Design review of the part built by this model. Coordinates are the model's own, in mm. Give positions to 0.01 mm unless a question says otherwise; leave off trailing zeros. Write each loop counter-clockwise with the first axis right and the second up, starting at its lowest first coordinate (ties: lowest second). Pieces come first, ordered by that corner, then holes. Notation, with made-up numbers: M 4.5,85 L 29.5,85 A13 cw 29.5,107 Z; hole C 60.25,54 d11. An arc over 180 degrees is marked long. Answer in a Markdown table with one row per item.
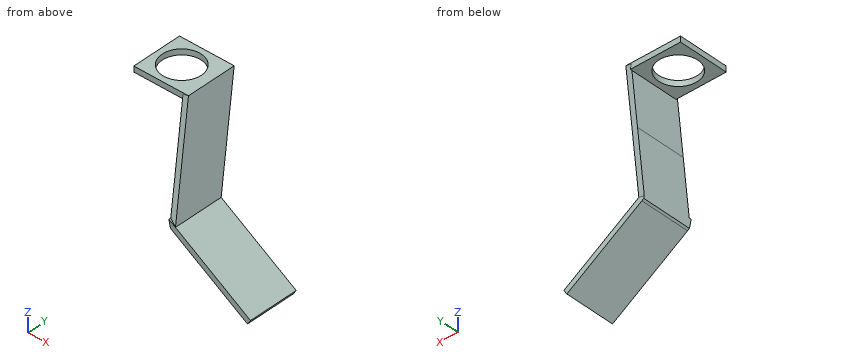
Autodesk Inventor part; units mm, degrees
ref_plane "YZ Plane" through (0, 0, 0) normal (1, 0, 0) x (0, 1, 0)
ref_plane "XZ Plane" through (0, 0, 0) normal (0, 1, 0) x (-1, 0, 0)
ref_plane "XY Plane" through (0, 0, 0) normal (0, 0, 1) x (1, 0, 0)
sketch "Sketch1" plane through (0, 0, 0) normal (0, 1, 0) x (-1, 0, 0)
  line L0 (43.0137, 64.3915) -> (32.1817, 14.8739)
  line L1 (-10.5502, -12.5966) -> (-8.8333, -15.2673)
  line L2 (-8.8333, -15.2673) -> (35.0028, 12.913)
  line L3 (35.0028, 12.913) -> (46.1153, 63.713)
  line L4 (46.1153, 63.713) -> (43.0137, 64.3915)
  line L5 (-10.5502, -12.5966) -> (-10.5502, 12.913)
  line L6 (-10.5502, -12.5966) -> (32.1817, 14.8739)
  line L7 (46.1153, 63.713) -> (74.6903, 63.713)
  line L8 (74.6903, 63.713) -> (74.6903, 66.888)
  line L9 (74.6903, 66.888) -> (43.5598, 66.888)
  line L10 (43.0137, 64.3915) -> (43.5598, 66.888)
  point P0 (0, 0)
  dimension "d0" = 3.175
  dimension "d1" = 3.175
  dimension "d3" = 50.8
  dimension "d4" = 57.265
  dimension "d5" = 50.8
  dimension "d6" = 11.1125
  dimension "d7" = 28.575
  dimension "d8" = 3.175
extrude "Extrusion1" add sketch "Sketch1" along normal blind 28.575
sketch "Sketch2" plane through (-74.6903, 0, 66.888) normal (0, 0, 1) x (1, 0, 0)
  line L0 (28.575, 0) -> (0, 0)
  line L1 (0, 0) -> (0, 28.575)
  line L2 (28.575, 28.575) -> (0, 28.575)
  line L3 (28.575, 0) -> (28.575, 28.575)
  line L4 (28.575, 28.575) -> (0, 28.575)
  line L5 (0, 0) -> (0, 28.575)
  circle A0 centre (14.2875, 14.2875) radius 11.1125
  point P0 (74.6903, 0)
  point P1 (14.2875, 28.575)
  point P2 (0, 14.2875)
  dimension "d11" = 22.225
extrude "Extrusion2" cut sketch "Sketch2" against normal blind 28.575 contours A0
sketch "Sketch3" plane through (10.5502, 0, -12.5966) normal (0.5408, 0, 0.8412) x (0.8412, 0, -0.5408)
  line L0 (-50.8, 0) -> (-50.8, 28.575)
  line L1 (-50.8, 7.9375) -> (0, 7.9375)
  line L2 (0, 7.9375) -> (0, -20.6375)
  line L3 (0, -20.6375) -> (-50.8, -20.6375)
  line L4 (-50.8, -20.6375) -> (-50.8, 7.9375)
  line L5 (-50.8, 28.575) -> (0, 28.575)
  point P0 (-15.6863, 0)
  dimension "d14" = 50.8
  dimension "d15" = 28.575
  dimension "d16" = 20.6375
sketch "Sketch4" plane through (-32.1817, 0, 14.8739) normal (0.9769, 0, 0.2137) x (0.2137, 0, -0.9769)
  line L0 (-53.2441, 0) -> (-53.2441, 28.575)
  line L1 (-53.2441, 28.575) -> (0, 7.9375)
  line L2 (0, 0) -> (0, 28.575)
  line L3 (0, 7.9375) -> (0, -20.6375)
  line L4 (0, -20.6375) -> (-53.2441, 0)
  line L5 (-53.2441, 28.575) -> (-53.2441, 0)
  point P0 (21.4074, 0)
  dimension "d17" = 20.6375
  dimension "d18" = 28.575
sketch "Sketch5" plane through (-32.1817, 0, 14.8739) normal (0.9769, 0, 0.2137) x (0.2137, 0, -0.9769)
  line L0 (-53.2441, 41.9678) -> (42.8737, 41.9678)
  line L1 (42.8737, 41.9678) -> (42.8737, -28.4609)
  line L2 (42.8737, -28.4609) -> (-53.2441, -28.4609)
  line L3 (-53.2441, -28.4609) -> (-53.2441, 41.9678)
  point P0 (21.4074, 0)
extrude "Extrusion3" cut sketch "Sketch5" along normal blind 50.8 and the other way blind 3.175
extrude "Extrusion4" add sketch "Sketch4" against normal blind 3.175
extrude "Extrusion5" add sketch "Sketch3" against normal blind 3.175
sketch "Sketch6" plane through (8.8333, 0, -15.2673) normal (-0.5408, 0, -0.8412) x (-0.8412, 0, 0.5408)
  line L0 (50.8, 7.9375) -> (0, 7.9375)
  line L1 (50.8, 7.9375) -> (63.8738, 7.9375)
  line L2 (63.8738, 7.9375) -> (63.8738, -20.6375)
  line L3 (63.8738, -20.6375) -> (50.8, -20.6375)
  line L4 (50.8, -20.6375) -> (50.8, 7.9375)
  point P0 (15.6863, 0)
extrude "Extrusion6" add sketch "Sketch6" against normal blind 3.175
sketch "Sketch7" plane through (-35.2833, 0, 14.1954) normal (-0.9769, 0, -0.2137) x (-0.2137, 0, 0.9769)
  line L0 (50.6885, 27.5845) -> (0, 7.9375)
  line L1 (3.1832, -19.4037) -> (53.2441, 0)
  line L2 (0, 7.9375) -> (3.1832, 7.9375)
  line L3 (0, 7.9375) -> (-56.9759, -14.1465)
  line L4 (-56.9759, -14.1465) -> (-50.1301, -40.068)
  line L5 (53.2441, 0) -> (0, -20.6375)
  line L6 (-50.1301, -40.068) -> (0, -20.6375)
  line L7 (0, 7.9375) -> (-35.9676, 7.9375)
  line L8 (0, 7.9375) -> (0, -20.6375)
  line L9 (11.5155, 12.4009) -> (21.1446, -12.4418)
  line L10 (-34.1585, 31.8696) -> (27.6424, 31.8696)
  line L11 (27.6424, 31.8696) -> (27.6424, -37.0154)
  line L12 (27.6424, -37.0154) -> (-34.1585, -37.0154)
  line L13 (-34.1585, -37.0154) -> (-34.1585, 31.8696)
  point P0 (-21.4074, 0)
extrude "Extrusion7" cut sketch "Sketch7" along normal blind 25.4 contours L9 L1 L5 L8 L0 | L0 L7 L13 L10 L11 | L0 L11 L1 L9 | L8 L6 L13 L3 | L3 L13 L7 | L1 L11 L12 L13 L6 L5
properties part number "Spinner to Top"
1) Add section B-B (x = -54). Write out the cut boundary in (y, z) (3 decimals).
Geometry says:
| item | result |
|---|---|
| outline | M 0,63.713 L 5.205,63.713 L 5.205,66.888 L 0,66.888 Z; M 23.37,63.713 L 28.575,63.713 L 28.575,66.888 L 23.37,66.888 Z |
2) Add section D-D (z = -2.5). Write out the cut boundary in (x, y).
Geometry says:
| item | result |
|---|---|
| outline | M -11.03,-20.64 L -5.15,-20.64 L -5.15,7.94 L -11.03,7.94 Z |
3) To check wall thickness, follow probe 1 along Z at (x, y) = (-51.5, 4); probe 2 along Y at (x, z) = (-22, 8); probe 3 along Z at (x, y) = (-28, 6.5). State the ranges of each line that lie inside material, in increasing order. Write a range as [from, to].
Geometry says:
| item | result |
|---|---|
| probe 1 | [63.71, 66.89] |
| probe 2 | [-20.64, 7.94] |
| probe 3 | [8.41, 12.19] |
4) Insertion check: P1, Ø10, axis at y = 8.5, z = 51, coming from the +X side; P2, Ø24, axis at x = -4.5, z = 6.5, coming from the +Y side; P3, Ø6, axis at y = -15, z = 22.5, coming from the +X side. Each pin has a flat end and moves straight along its axis. Give the tip position at first contact, or say it passes through.
Geometry says:
| item | result |
|---|---|
| P1 | x = -38.99 |
| P2 | y = 7.94 |
| P3 | x = -33.19 |
